```python
from build123d import *

# Parameters (mm, degrees)
BOSS_EXTRUDE1_DEPTH = 75
CUT_EXTRUDE1_DEPTH  = 8.2
CUT_EXTRUDE2_DEPTH  = 15
FILLET1_R           = 3
SKETCH5_R           = 4
CUT_EXTRUDE3_DEPTH  = 9
CUT_EXTRUDE4_REACH  = 47
SKETCH6_R           = 3
CUT_EXTRUDE5_REACH  = 36
SKETCH7_R           = 3
CUT_EXTRUDE7_REACH  = 47
SKETCH10_R          = 2.5
CUT_EXTRUDE8_REACH  = 68
SKETCH11_R          = 3
CUT_EXTRUDE10_DEPTH = 2
FILLET3_R           = 2
CUT_EXTRUDE11_DEPTH = 12
CUT_EXTRUDE12_REACH = 47
SKETCH16_R          = 1.75
SKETCH17_R          = 1
CUT_EXTRUDE13_DEPTH = 5
SKETCH8_R           = 7.5
CUT_EXTRUDE14_DEPTH = 60


with BuildPart() as part:
    # Sketch1 → Boss-Extrude1 (new body)
    with BuildSketch(Plane(origin=(0, 0, 0), x_dir=(0, 0, -1), z_dir=(1, 0, 0))):
        Polygon((24, 0), (34, 10), (34, 45), (0, 45), (0, 0), align=None)
    extrude(amount=-BOSS_EXTRUDE1_DEPTH)

    # Sketch2 → Cut-Extrude1 (cut)
    with BuildSketch(Plane(origin=(0, 0, 0), x_dir=(0, 0, -1), z_dir=(1, 0, 0))):
        with BuildLine():
            Line((19, 0), (16.821625926, 12.584303175))
            ThreePointArc((16.821625926, 12.584303175), (17.294620228, 17.084983398), (20.058295206, 20.668549597))
            Line((20.058295206, 20.668549597), (34, 31))
            Line((34, 31), (34, 0))
            Line((34, 0), (19, 0))
        make_face()
    extrude(amount=-CUT_EXTRUDE1_DEPTH, mode=Mode.SUBTRACT)

    # Sketch3 → Cut-Extrude2 (cut)
    with BuildSketch(Plane(origin=(0, 0, -34), x_dir=(-1, 0, 0), z_dir=(0, 0, -1))):
        Polygon((31, 45), (31, 31), (61, 31), (47, 45), align=None)
    extrude(amount=-CUT_EXTRUDE2_DEPTH, mode=Mode.SUBTRACT)

    # Fillet1
    fillet1_edges = [part.edges().sort_by_distance(p)[0] for p in [
        (-61, 31, -26.5),
        (-31, 31, -26.5),
    ]]
    fillet(fillet1_edges, radius=FILLET1_R)

    # Sketch5 → Cut-Extrude3 (cut)
    with BuildSketch(Plane(origin=(0, 0, 0), x_dir=(0, 0, -1), z_dir=(1, 0, 0))):
        with Locations((28.5, 39)):
            Circle(SKETCH5_R)
    extrude(amount=-CUT_EXTRUDE3_DEPTH, mode=Mode.SUBTRACT)

    # Sketch6 → Cut-Extrude4 (cut, up to next)
    with BuildSketch(Plane(origin=(0, 45, 0), x_dir=(1, 0, 0), z_dir=(0, 1, 0)), mode=Mode.PRIVATE) as cut_extrude4_sk1:
        with Locations((-4.5, 29.5)):
            Circle(SKETCH6_R)
    cut_extrude4_tool1 = extrude(cut_extrude4_sk1.sketch, amount=-CUT_EXTRUDE4_REACH, mode=Mode.PRIVATE) & part.part
    add(cut_extrude4_tool1.solids().sort_by_distance((-4.5, 45, -29.5))[0], mode=Mode.SUBTRACT)

    # Sketch7 → Cut-Extrude5 (cut, up to next)
    with BuildSketch(Plane.XY, mode=Mode.PRIVATE) as cut_extrude5_sk1:
        with Locations((-5, 5)):
            Circle(SKETCH7_R)
    cut_extrude5_tool1 = extrude(cut_extrude5_sk1.sketch, amount=-CUT_EXTRUDE5_REACH, mode=Mode.PRIVATE) & part.part
    add(cut_extrude5_tool1.solids().sort_by_distance((-5, 5, 0))[0], mode=Mode.SUBTRACT)

    # Sketch10 → Cut-Extrude7 (cut, up to next)
    with BuildSketch(Plane(origin=(0, 45, 0), x_dir=(1, 0, 0), z_dir=(0, 1, 0)), mode=Mode.PRIVATE) as cut_extrude7_sk1:
        with Locations((-4.5, 29.5)):
            Circle(SKETCH10_R)
    cut_extrude7_tool1 = extrude(cut_extrude7_sk1.sketch, amount=-CUT_EXTRUDE7_REACH, mode=Mode.PRIVATE) & part.part
    add(cut_extrude7_tool1.solids().sort_by_distance((-4.5, 45, -29.5))[0], mode=Mode.SUBTRACT)

    # Sketch11 → Cut-Extrude8 (cut, up to next)
    with BuildSketch(Plane(origin=(-9, 0, 0), x_dir=(0, 0, -1), z_dir=(1, 0, 0)), mode=Mode.PRIVATE) as cut_extrude8_sk1:
        with Locations((28.5, 39)):
            Circle(SKETCH11_R)
    cut_extrude8_tool1 = extrude(cut_extrude8_sk1.sketch, amount=-CUT_EXTRUDE8_REACH, mode=Mode.PRIVATE) & part.part
    add(cut_extrude8_tool1.solids().sort_by_distance((-9, 39, -28.5))[0], mode=Mode.SUBTRACT)

    # Sketch13 → Cut-Extrude10 (cut)
    with BuildSketch(Plane.XY):
        Polygon((-74, 44), (-74, 1), (-10, 1), (-10, 10), (-1, 10), (-1, 44), align=None)
    extrude(amount=-CUT_EXTRUDE10_DEPTH, mode=Mode.SUBTRACT)

    # Fillet3
    fillet3_edges = [part.edges().sort_by_distance(p)[0] for p in [
        (-74, 44, -1),
        (-1, 44, -1),
        (-1, 10, -1),
        (-10, 10, -1),
        (-10, 1, -1),
        (-74, 1, -1),
    ]]
    fillet(fillet3_edges, radius=FILLET3_R)

    # Sketch14 → Cut-Extrude11 (cut)
    with BuildSketch(Plane.XY.offset(-2)):
        with BuildLine():
            ThreePointArc((-6.458039892, 12), (-5.621320344, 14.621320344), (-3, 15.458039892))
            Line((-3, 15.458039892), (-3, 38.541960108))
            ThreePointArc((-3, 38.541960108), (-5.621320344, 39.378679656), (-6.458039892, 42))
            Line((-6.458039892, 42), (-68.541960108, 42))
            ThreePointArc((-68.541960108, 42), (-68.510508432, 41.750878781), (-68.5, 41.5))
            ThreePointArc((-68.5, 41.5), (-69.563508327, 39.208712153), (-72, 38.541960108))
            Line((-72, 38.541960108), (-72, 6.458039892))
            ThreePointArc((-72, 6.458039892), (-69.563508327, 5.791287847), (-68.5, 3.5))
            ThreePointArc((-68.5, 3.5), (-68.510508432, 3.249121219), (-68.541960108, 3))
            Line((-68.541960108, 3), (-12, 3))
            Line((-12, 3), (-12, 8))
            ThreePointArc((-12, 8), (-10.828427125, 10.828427125), (-8, 12))
            Line((-8, 12), (-6.458039892, 12))
        make_face()
    extrude(amount=-CUT_EXTRUDE11_DEPTH, mode=Mode.SUBTRACT)

    # Sketch16 → Cut-Extrude12 (cut, up to next)
    with BuildSketch(Plane.XZ, mode=Mode.PRIVATE) as cut_extrude12_sk1:
        with Locations((-69, -11.25)):
            Circle(SKETCH16_R)
    cut_extrude12_tool1 = extrude(cut_extrude12_sk1.sketch, amount=-CUT_EXTRUDE12_REACH, mode=Mode.PRIVATE) & part.part
    add(cut_extrude12_tool1.solids().sort_by_distance((-69, 0, -11.25))[0], mode=Mode.SUBTRACT)
    # Sketch16 → Cut-Extrude12 (cut, up to next)
    with BuildSketch(Plane.XZ, mode=Mode.PRIVATE) as cut_extrude12_sk2:
        with Locations((-65, -11.25)):
            Circle(SKETCH16_R)
    cut_extrude12_tool2 = extrude(cut_extrude12_sk2.sketch, amount=-CUT_EXTRUDE12_REACH, mode=Mode.PRIVATE) & part.part
    add(cut_extrude12_tool2.solids().sort_by_distance((-65, 0, -11.25))[0], mode=Mode.SUBTRACT)
    # Sketch16 → Cut-Extrude12 (cut, up to next)
    with BuildSketch(Plane.XZ, mode=Mode.PRIVATE) as cut_extrude12_sk3:
        with Locations((-61, -11.25)):
            Circle(SKETCH16_R)
    cut_extrude12_tool3 = extrude(cut_extrude12_sk3.sketch, amount=-CUT_EXTRUDE12_REACH, mode=Mode.PRIVATE) & part.part
    add(cut_extrude12_tool3.solids().sort_by_distance((-61, 0, -11.25))[0], mode=Mode.SUBTRACT)

    # Sketch17 → Cut-Extrude13 (cut)
    with BuildSketch(Plane.XY.offset(-2)):
        with Locations((-71.5, 41.5)):
            Circle(SKETCH17_R)
        with Locations((-71.5, 3.5)):
            Circle(SKETCH17_R)
        with Locations((-3.5, 12.5)):
            Circle(SKETCH17_R)
        with Locations((-3.5, 41.5)):
            Circle(SKETCH17_R)
    extrude(amount=-CUT_EXTRUDE13_DEPTH, mode=Mode.SUBTRACT)

    # Sketch8 → Cut-Extrude14 (cut)
    with BuildSketch(Plane(origin=(-8.2, 0, 0), x_dir=(0, 0, -1), z_dir=(1, 0, 0))):
        with Locations((25, 14)):
            Circle(SKETCH8_R)
    extrude(amount=-CUT_EXTRUDE14_DEPTH, mode=Mode.SUBTRACT)


solid = part.part
```
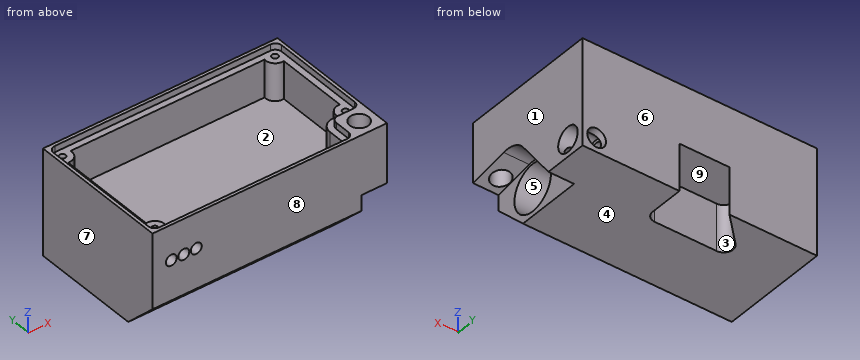
Geometry: final body of the model. Coordinates: model frame, mm. Face numbers are marked on the shaded views. A direction names the side the tool comes from. Coordinates: 2 decimals unless noted, no trailing zeros. Order: outer loops, then holes, each group sorted by start corner. A loop starts at its lowest first (then second) coordinate and runs counter-clockwise, first axis right, second up. Notation, with made-up numbers: (40.25, -1) - (72.25, -1) arc R14 cw to (72.25, 7) - close; hole circle Ø4 at (-7.5, 54). An arc over 180 degrees is marked (long way). Return JSON: item names as keys, results as strings. Group by question number.
1. Set-up query: the marked faces 1, 2, 3, 4 and 5. Return all of +Z, -Z, +X, -X, +Y, -Y with unobstructed straight access to the full face (end or side cutting, diameter ignored); none if empty.
2. Pull-direction query (Y, two-part tool) for the marked faces 6, 7, 8 and 9; classes: pulls with the +Y half, pulls with the -Y half, needs draft (parallel to the pull), parting line crosses it, or undercut.
3. Cut plane C-C (y = 19). Output: boundary loops of the cut face in (x, z).
4. Cut plane B-B (x = -27.5). Output: boundary loops of the cut face in (y, z).
5. Pin query (flat end, axial travel): pin 1 (3 mm diameter, centred on x = -64, y = 33.5, fed in from +Z); pin 2 (2 mm diameter, centred on x = -69, z = -11.25, fed in from -Y); pin 3 (7.5 mm diameter, centred on y = 10.5, z = -22.5, fed in from +X). Return the tip coordinate at first contact, or that it passes through.
6. Cut plane A-A (x = -65). Output: boundary loops of the cut face in (y, z), plus the area to 3 significant figures.
7. Material intervals for line 1 along X through (y, z) = (1, -11); line 2 along Y through (x, z) = (-71.5, -5.6); line 3 along Y through (x, z) = (-25.25, -28.5), sorted ascending. Write a range as [from, to].
Resolved:
{
 "1": {"face 1": "+Z, -Z, +X, +Y, -Y", "face 2": "+Z", "face 3": "-Z", "face 4": "-Z, +X, -X, +Y, -Y", "face 5": "+X"},
 "2": {"face 6": "pulls with the +Y half", "face 7": "needs draft", "face 8": "pulls with the -Y half", "face 9": "undercut"},
 "3": {"outline": "(-75, -34) - (-8.2, -34) - (-8.2, -30.59) - (-68.2, -30.59) - (-68.2, -19.41) - (-8.2, -19.41) - (-8.2, -18.38) - (0, -18.38) - (0, 0) - (-1, 0) - (-1, -2) - (-3, -2) - (-3, -14) - (-72, -14) - (-72, -2) - (-74, -2) - (-74, 0) - (-75, 0) - close"},
 "4": {"outline": "(0, -24) - (10, -34) - (45, -34) - (45, 0) - (44, 0) - (44, -2) - (42, -2) - (42, -14) - (3, -14) - (3, -2) - (1, -2) - (1, 0) - (0, 0) - close; hole circle Ø15 at (14, -25); hole circle Ø6 at (39, -28.5)"},
 "5": {"pin 1": "stops at z = -14", "pin 2": "stops at y = 38.9", "pin 3": "stops at x = -8.2"},
 "6": {"outline": "(0, -24) - (10, -34) - (45, -34) - (45, 0) - (44, 0) - (44, -2) - (42, -2) - (42, -14) - (3, -14) - (3, -13) - (0, -13) - close; (0, -9.5) - (3, -9.5) - (3, -2) - (1, -2) - (1, 0) - (0, 0) - close; hole circle Ø15 at (14, -25)", "area": "739 mm²"},
 "7": {"line 1": "x = [-75, -70.73], [-67.27, -66.73], [-63.27, -62.73], [-59.27, 0]", "line 2": "y = [0, 2.5], [4.5, 6.5], [38.5, 40.5], [42.5, 45]", "line 3": "y = [4.5, 7.37], [20.63, 36], [42, 45]"}
}
